Geometry check sheet. Reference: the model listing, model coordinates, mm. A direction names the side the tool comes from. Coordinates: 2 decimals unless noted, no trailing zeros. Write each loop counter-clockwise with the first axis right and the second up, starting at its lowest first coordinate (ties: lowest second). Pieces come first, ordered by that corner, then holes. Notation, with made-up numbers: (56, 12) -> (92, 12) arc R27 cw to (92, 44) -> close; hole circle Ø4 at (47.25, -8). An arc over 180 degrees is marked (long way). Use a Markdown table: item, result.
```python
from build123d import *

# Parameters (mm, degrees)
F0_W     = 3.05
F0_H     = 20
F1_DEPTH = 3


with BuildPart() as f1:
    # F0 (on Top) → F1 (new body)
    with BuildSketch(Plane.XY):
        with Locations((22.525, 0)):
            Rectangle(F0_W, F0_H)
        Polygon((9.95, -38), (21, -38), (21, -10), (21, 10), (21, 38), (9.95, 38), (9.95, 34.95), (-9.95, 34.95), (-9.95, 38), (-21, 38), (-21, -38), (-9.95, -38), (-9.95, -34.95), (9.95, -34.95), align=None)
    extrude(amount=F1_DEPTH)


solid = f1.part
```
Item 1: Depth check by flat-ended pin: P1, Ø1.5, axis at y = 37, z = 1, coming from the +X side; P2, Ø1.5, axis at x = -3, z = 1, coming from the +Y side. Enter the tip coordinate at first touch or a pass-through.
Answer block:
| item | result |
|---|---|
| P1 | stops at x = 21 |
| P2 | stops at y = 34.95 |
Item 2: Section check A-A on z = 2.2. Record the boundary of the cut face in (x, y), then the cut area to 3 significant figures.
Answer block:
| item | result |
|---|---|
| outline | (-21, -38) -> (-9.95, -38) -> (-9.95, -34.95) -> (9.95, -34.95) -> (9.95, -38) -> (21, -38) -> (21, -10) -> (24.05, -10) -> (24.05, 10) -> (21, 10) -> (21, 38) -> (9.95, 38) -> (9.95, 34.95) -> (-9.95, 34.95) -> (-9.95, 38) -> (-21, 38) -> close |
| area | 3,130 mm^2 |
Item 3: Section check B-B on x = 1.5. Record the boundary of the cut face in (y, z).
Answer block:
| item | result |
|---|---|
| outline | (-34.95, 0) -> (34.95, 0) -> (34.95, 3) -> (-34.95, 3) -> close |
Item 4: Section check C-C on y = 26. Record the boundary of the cut face in (x, z).
Answer block:
| item | result |
|---|---|
| outline | (-21, 0) -> (21, 0) -> (21, 3) -> (-21, 3) -> close |
Item 5: Tool access check on faces 5 (the flat face through (23, 10, 1)), 6 (the flat face through (-9.95, -36, 1)), 7 (the flat face through (21, -24, 1)), 8 (the flat face through (0, 34.95, 1)). Record the directions out of +Z, -Z, +X, -X, +Y, -Y that give a thin tool (end or side, any length) a straight path to the whole face; none if there is none.
Answer block:
| item | result |
|---|---|
| face 5 | +Z, -Z, +X, +Y |
| face 6 | +Z, -Z, -Y |
| face 7 | +Z, -Z, +X, -Y |
| face 8 | +Z, -Z, +Y |
Item 6: Thickness scan on L1, parallel to X at y = 30, z = 1.25; L2, parallel to Y at x = 3, z = 1.9. Record the ranges inside material, lowest first. Write a range as [from, to].
Answer block:
| item | result |
|---|---|
| L1 | x = [-21, 21] |
| L2 | y = [-34.95, 34.95] |
Item 7: Mould release check, pull along X, two halves, no side actions. Record for faces 1 (the flat face through (21, 24, 1)), 2 (the flat face through (9.95, -36, 1)), 3 (the flat face through (1, 1, 0)), 4 (the flat face through (-21, 1, 1)): +X half, -X half, draft (parallel to the pull), parting line (faces both ways), or undercut.
Answer block:
| item | result |
|---|---|
| face 1 | +X half |
| face 2 | undercut |
| face 3 | draft |
| face 4 | -X half |
